Input: part model. Units: mm. Frame: model coordinates. A direction names the side the tool comes from. Give positions to 0.01 mm unless a question says otherwise; leave off trailing zeros. Write each loop counter-clockwise with the first axis right and the second up, starting at its lowest first coordinate (ties: lowest second). Pieces come first, ordered by that corner, then holes. Notation, with made-up numbers: (67.5, 21.5) - (90.5, 21.5) arc R24 ccw to (90.5, 47.5) - close; hole circle Ø11 at (72, -8). An arc over 180 degrees is marked (long way). Answer as CSV lines item,"result".
```python
from build123d import *

# Parameters (mm, degrees)
EXTRUDE_1_DEPTH     = 190
SKETCH_2_R          = 2.25
CUT_EXTRUDE_1_DEPTH = 2
SKETCH1_R           = 1.6
CUT_EXTRUDE1_DEPTH  = 2


with BuildPart() as part:
    # Эскиз1 → Бобышка-Вытянуть1 (new body)
    with BuildSketch(Plane(origin=(0, 0, 0), x_dir=(1, 0, 0), z_dir=(0, 1, 0))):
        Polygon((0, 0), (0, 20), (1, 20), (1, 1), (20, 1), (20, 0), align=None)
    extrude(amount=EXTRUDE_1_DEPTH)

    # Эскиз2 → Вырез-Вытянуть1 (cut, through all)
    with BuildSketch(Plane(origin=(0, 0, -1), x_dir=(-1, 0, 0), z_dir=(0, 0, -1))):
        with Locations((-10.5, 10)):
            Circle(SKETCH_2_R)
        with Locations((-10.5, 180)):
            Circle(SKETCH_2_R)
    extrude(amount=-CUT_EXTRUDE_1_DEPTH, mode=Mode.SUBTRACT)

    # Sketch1 → Cut-Extrude1 (cut, through all)
    with BuildSketch(Plane(origin=(1, 0, 0), x_dir=(0, 0, -1), z_dir=(1, 0, 0))):
        with Locations((7, 155)):
            Circle(SKETCH1_R)
        with Locations((7, 122)):
            Circle(SKETCH1_R)
    extrude(amount=-CUT_EXTRUDE1_DEPTH, mode=Mode.SUBTRACT)


solid = part.part
```
Item 1: Cut plane A-A on y = 155. Return the cut outline in (x, z), plus the area to 3 significant figures.
The answers:
outline,"(0, -20) - (1, -20) - (1, -8.6) - (0, -8.6) - close; (0, -5.4) - (1, -5.4) - (1, -1) - (20, -1) - (20, 0) - (0, 0) - close"
area,"35.8 mm²"
Item 2: Mould query, pull axis Y, two halves, no side actions, for faces 3 (the face through (5.6, 190, -0.4)), 4 (the face through (5.6, 0, -0.4)), 5 (the face through (0.51, 120.44, -6.65)). Classes: +Y half, -Y half, draft (parallel to the pull), parting line (faces both ways), or undercut.
The answers:
face 3,"+Y half"
face 4,"-Y half"
face 5,"undercut"
Item 3: Cut plane C-C on y = 180. Return the cut outline in (x, z), plus the area to 3 significant figures.
The answers:
outline,"(0, -20) - (1, -20) - (1, -1) - (8.25, -1) - (8.25, 0) - (0, 0) - close; (12.75, -1) - (20, -1) - (20, 0) - (12.75, 0) - close"
area,"34.5 mm²"
Item 4: Reachability of faces 1 (the face through (1, 94, -11)), 2 (the face through (10, 94, 0)) from +Z, -Z, +X, -X, +Y, -Y: full face, straight path, thin tool, end or side. Return the list, or none.
The answers:
face 1,"-Z, +X, +Y, -Y"
face 2,"+Z, +X, -X, +Y, -Y"
Item 5: Cut plane B-B on x = 10.5. Return the cut outline in (y, z), plus the area to 3 significant figures.
The answers:
outline,"(0, -1) - (7.75, -1) - (7.75, 0) - (0, 0) - close; (12.25, -1) - (177.75, -1) - (177.75, 0) - (12.25, 0) - close; (182.25, -1) - (190, -1) - (190, 0) - (182.25, 0) - close"
area,"181 mm²"
Item 6: Contact query for flat-ended pins moving along their axis: pin 1 (5 mm diameter, centred on x = 10.5, y = 180, fed in from -Z); pin 2 (5 mm diameter, centred on y = 66, z = -4.5, fed in from +X). Output: stop coordinate, or through.
The answers:
pin 1,"z = -1"
pin 2,"x = 1"
Item 7: Ray query, line 1 (Y direction, x = 0.45, z = -7); line 2 (Y direction, x = 10.5, z = -0.3); line 3 (Z direction, x = 0.35, y = 155). Return the intervals inside material, ascending. Write a range as from..to.
The answers:
line 1,"0..120.4, 123.6..153.4, 156.6..190"
line 2,"0..7.75, 12.25..177.75, 182.25..190"
line 3,"-20..-8.6, -5.4..0"
Item 8: Cut plane D-D on z = -15.25. Return the cut outline in (x, y), plus the area to 3 significant figures.
The answers:
outline,"(0, 0) - (1, 0) - (1, 190) - (0, 190) - close"
area,"190 mm²"
